from build123d import *

# Parameters (mm, degrees)
SKETCH1_R             = 18
BOSS_EXTRUDE1_DEPTH   = 2
SKETCH2_R             = 1.6
CUT_EXTRUDE1_DEPTH    = 2
F_2_0MM_DOWEL_HOLE1_D = 2
SKETCH_1_R            = 10
CUT_EXTRUDE_1_DEPTH   = 39.942264957


with BuildPart() as part:
    # Sketch1 → Boss-Extrude1 (new body)
    with BuildSketch(Plane.XY):
        with BuildLine():
            ThreePointArc((-27.5, 0), (0, -27.5), (27.5, 0))
            ThreePointArc((27.5, 0), (0, 27.5), (-27.5, 0))
        make_face()
        Circle(SKETCH1_R, mode=Mode.SUBTRACT)
    extrude(amount=BOSS_EXTRUDE1_DEPTH)

    # Sketch2 → Cut-Extrude1 (cut)
    with BuildSketch(Plane.XY.offset(2)):
        with Locations((0, 25.980762114)):
            Circle(SKETCH2_R)
        with Locations((-22.5, -12.990381057)):
            Circle(SKETCH2_R)
        with Locations((22.5, -12.990381057)):
            Circle(SKETCH2_R)
    extrude(amount=-CUT_EXTRUDE1_DEPTH, mode=Mode.SUBTRACT)

    # Ø2.0mm Dowel Hole1 (through all)
    with Locations(Plane(origin=(-19, 19, 2), x_dir=(1, 0, 0), z_dir=(0, 0, 1))):
        with Locations((0, 0), (2, -2), (36, -2), (38, 0), (36, -36), (38, -38), (0, -38), (2, -36)):
            Hole(F_2_0MM_DOWEL_HOLE1_D / 2)

    # 스케치1 → 컷-돌출1 (cut, through all)
    with BuildSketch(Plane.XY):
        with Locations((-34, 0)):
            Circle(SKETCH_1_R)
        with Locations((34, 0)):
            Circle(SKETCH_1_R)
    extrude(amount=CUT_EXTRUDE_1_DEPTH, mode=Mode.SUBTRACT)


solid = part.part
Work out the finished part from the listing and answer in its coordinate system (mm). Round coordinates to 2 decimals unless told otherwise and drop trailing zeros. Order: outer loops, then holes, each group sorted by start corner. A loop starts at its lowest first (then second) coordinate and runs counter-clockwise, first axis right, second up. Notation, with made-up numbers: M 24,3 L 60,3 A6 cw 60,14 Z; hole C 54.25,87.5 d3. An arc over 180 degrees is marked long. One line per item, written item: value.
Q1. Find section A-A on x = -17. Write down the section's boundary in (y, z).
Derived:
outline: M -21.62,0 L -18,0 L -18,2 L -21.62,2 Z; M -16,0 L -5.92,0 L -5.92,2 L -16,2 Z; M 5.92,0 L 16,0 L 16,2 L 5.92,2 Z; M 18,0 L 21.62,0 L 21.62,2 L 18,2 Z
Q2. Determine the mould class of faces 1 (the face through (18.271, -18.315, 0.986)), 2 (the face through (-21.924, -16.601, 0.986)), 3 (the face through (17.4, -5.7, 2)) for opening direction Y: released by +Y, released by -Y, zero draft, split by the parting line, or undercut.
Derived:
face 1: undercut
face 2: released by -Y
face 3: zero draft
Q3. Find section D-D on x = 12. Write down the section's boundary in (y, z), then the cut area to 3 significant figures.
Derived:
outline: M -24.74,0 L -13.42,0 L -13.42,2 L -24.74,2 Z; M 13.42,0 L 24.74,0 L 24.74,2 L 13.42,2 Z
area: 45.3 mm²
Q4. Find section C-C on z = 1.3. Write down the section's boundary in (x, y).
Derived:
outline: M -26.65,-6.78 A27.5 ccw -24.07,-13.3 A1.6 cw long -23.55,-14.19 A27.5 ccw -19.99,-18.88 A1 cw long -18.88,-19.99 A27.5 ccw 18.88,-19.99 A1 cw long 19.99,-18.88 A27.5 ccw 23.55,-14.19 A1.6 cw long 24.07,-13.3 A27.5 ccw 26.65,-6.78 A10 cw 26.65,6.78 A27.5 ccw 19.99,18.88 A1 cw long 18.88,19.99 A27.5 ccw 0.52,27.5 A1.6 cw long -0.52,27.5 A27.5 ccw -18.88,19.99 A1 cw long -19.99,18.88 A27.5 ccw -26.65,6.78 A10 cw Z; hole C -17,-17 d2; hole C 0,0 d36; hole C -17,17 d2; hole C 17,-17 d2; hole C 17,17 d2
Q5. A flat-ended cylindrical pin translates along its axis: pin 1 (1 mm diameter, centred on x = -1.5, z = 1, fed in from +Y). Find the tip coordinate at first contact, or state that the pin passes through.
Derived:
pin 1: y = 27.48
Q6. Straight lines are drawn through the part: line 1 (Y direction, x = -5, z = 1.25); line 2 (X direction, y = 3, z = 0.6); line 3 (Y direction, x = -7, z = 1.75). For each, find the intervals that lie inside material, in ascending order.
Derived:
line 1: -27.04 to -17.29, 17.29 to 27.04
line 2: -24.46 to -17.75, 17.75 to 24.46
line 3: -26.59 to -16.58, 16.58 to 26.59
